Here's how the part is built. I have some questions about the finished solid (model axes, mm). A direction names the side the tool comes from. Round coordinates to 2 decimals unless told otherwise and drop trailing zeros. Loops run counter-clockwise (first coordinate to the right, second up) from the corner with the lowest first, then second, coordinate; pieces in that order, holes last. Notation, with made-up numbers: M 33.25,-18.75 L 71.25,-18.75 A21 ccw 71.25,9.25 Z; hole C 63,61 d2. An arc over 180 degrees is marked long. Answer as a JSON object with one key per item and string values.
from build123d import *

# Parameters (mm, degrees)
SKETCH2_W           = 66.675
SKETCH2_H           = 30.48
SKETCH2_R           = 3.175
BOSS_EXTRUDE2_DEPTH = 6.35


with BuildPart() as part:
    # Sketch2 → Boss-Extrude2 (new body)
    with BuildSketch(Plane.XY):
        with Locations((-20.6375, 0)):
            Rectangle(SKETCH2_W, SKETCH2_H)
        with Locations((-47.625, 0)):
            Circle(SKETCH2_R, mode=Mode.SUBTRACT)
        Polygon((3.666174209, 6.35), (-3.666174209, 6.35), (-7.332348419, 0), (-3.666174209, -6.35), (3.666174209, -6.35), (7.332348419, 0), align=None, mode=Mode.SUBTRACT)
    extrude(amount=BOSS_EXTRUDE2_DEPTH)


solid = part.part
Item 1: I want a section at B-B, the plane y = -1.5. Please give me the cut outline in (x, z) (3 decimals).
Resolved:
{"outline": "M -53.975,0 L -50.423,0 L -50.423,6.35 L -53.975,6.35 Z; M -44.827,0 L -6.466,0 L -6.466,6.35 L -44.827,6.35 Z; M 6.466,0 L 12.7,0 L 12.7,6.35 L 6.466,6.35 Z"}
Item 2: I want a section at C-C, the plane y = 2.5. Please give me the cut outline in (x, z) (3 decimals), then the cut area to 3 significant figures.
Resolved:
{"outline": "M -53.975,0 L -49.582,0 L -49.582,6.35 L -53.975,6.35 Z; M -45.668,0 L -5.889,0 L -5.889,6.35 L -45.668,6.35 Z; M 5.889,0 L 12.7,0 L 12.7,6.35 L 5.889,6.35 Z", "area": "324 mm²"}
Item 3: On a 3-axis mill with a long thin cutter (end or side, diameter ignored), from which of +Z, -Z, +X, -X, +Y, -Y can I reach the whole of each face in a straight line? I mean faces 4 (the face through (5.474, -3.219, 3.131)), 5 (the face through (12.7, 0, 3)). Say none if no direction works.
Resolved:
{"face 4": "+Z, -Z", "face 5": "+Z, -Z, +X, +Y, -Y"}
Item 4: If we mould it in two halves opening along Y, with no side actions, what happens to faces 1 (the face through (-5.474, 3.219, 3.131)), 2 (the face through (-21, -15.24, 3)), 3 (the face through (-21, 0, 6.35))? For each: pulls with the +Y half, pulls with the -Y half, needs draft (parallel to the pull), parting line crosses it, or undercut.
Resolved:
{"face 1": "undercut", "face 2": "pulls with the -Y half", "face 3": "needs draft"}
Item 5: I want a section at A-A, the plane z = 5.5. Please give me the cut outline in (x, y) (3 decimals).
Resolved:
{"outline": "M -53.975,-15.24 L 12.7,-15.24 L 12.7,15.24 L -53.975,15.24 Z; hole C -47.625,0 d6.35; hole M -7.332,0 L -3.666,-6.35 L 3.666,-6.35 L 7.332,0 L 3.666,6.35 L -3.666,6.35 Z"}
Item 6: Please list where these lines run through material, in increasing order: probe 1 along Y at (x, z) = (-50.5, 2.75); probe 2 along Y at (x, z) = (-6, 4.25); probe 3 along X at (y, z) = (-5, 5.5) (3 decimals). Write a range as from..to.
Resolved:
{"probe 1": "-15.24..-1.35, 1.35..15.24", "probe 2": "-15.24..-2.31, 2.31..15.24", "probe 3": "-53.975..-4.446, 4.446..12.7"}
